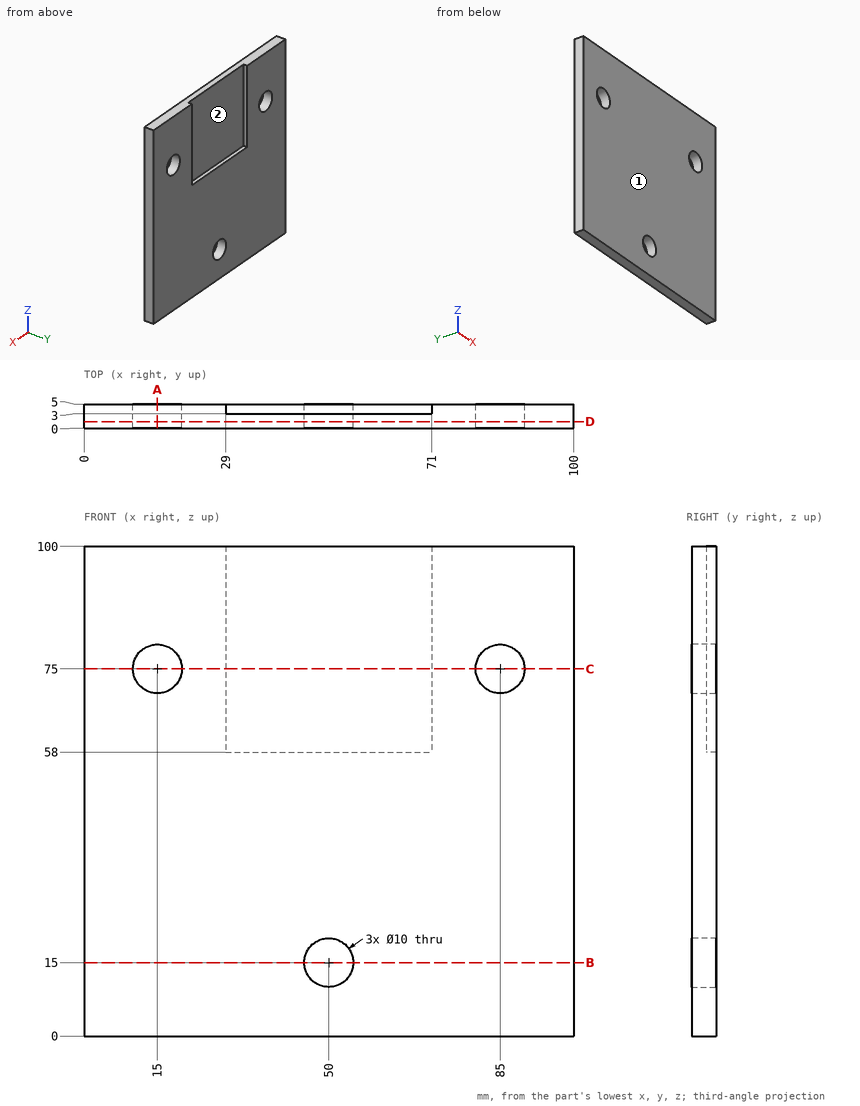
For this review, use the dimensioned drawing (mm, ordinates from the lowest corner) and the shaded views. Give positions to 0.01 mm unless a question says otherwise; leave off trailing zeros. Order: outer loops, then holes, each group sorted by start corner. A loop starts at its lowest first (then second) coordinate and runs counter-clockwise, first axis right, second up. Notation, with made-up numbers: (-38, -28) - (-3, -28) arc R12 ccw to (-3, -20) - close; hole circle Ø8 at (-9, 84). An arc over 180 degrees is marked (long way). Use CSV: the item, a comma, the result in double quotes. Start each with the question number.
Q1. Take a section at D-D (y = 1.4). State the section outline as (x, z) points, and give its area (3 significant figures).
Q2. Take a section at C-C (z = 75). State the section outline as (x, y) points, and give its area (3 significant figures).
Q3. Take a section at B-B (z = 15). State the section outline as (x, y) points, and give its area (3 significant figures).
Q4. For P1, Ø11.5, axis at x = 50, z = 15, coming from the -Y side; P2, Ø8, axis at x = 15, z = 75, coming from the -Y side; P3, Ø5, axis at x = 50.5, z = 65.5, coming from the +Y side; P4, Ø2, axis at x = 42, y = 4.5, coming from the +Z side, all flat-tipped, find the tip position at first contact; note any pin that passes through.
Q5. For line 1 (X direction, y = 1.3, z = 75); line 2 (X direction, y = 2.1, z = 15); line 3 (Y direction, x = 60, z = 76), list the stretches that pass through material, from the lowest coordinate up.
Q6. Take a section at A-A (x = 15). State the section outline as (y, z) points.
Q7. Draft analysis for pull direction X (two halves, no side actions). For the marked faces 1 and 2, state which applies: pulls with the +X half, pulls with the -X half, needs draft (parallel to the pull), parting line crosses it, or undercut.
Calculated:
1,outline,"(0, 0) - (100, 0) - (100, 100) - (0, 100) - close; hole circle Ø10 at (15, 75); hole circle Ø10 at (50, 15); hole circle Ø10 at (85, 75)"
1,area,"9,760 mm²"
2,outline,"(0, 0) - (10, 0) - (10, 5) - (0, 5) - close; (20, 0) - (80, 0) - (80, 5) - (71, 5) - (71, 3) - (29, 3) - (29, 5) - (20, 5) - close; (90, 0) - (100, 0) - (100, 5) - (90, 5) - close"
2,area,"316 mm²"
3,outline,"(0, 0) - (45, 0) - (45, 5) - (0, 5) - close; (55, 0) - (100, 0) - (100, 5) - (55, 5) - close"
3,area,"450 mm²"
4,P1,"stops at y = 0"
4,P2,"passes through"
4,P3,"stops at y = 3"
4,P4,"stops at z = 58"
5,line 1,"x = 0 to 10, 20 to 80, 90 to 100"
5,line 2,"x = 0 to 45, 55 to 100"
5,line 3,"y = 0 to 3"
6,outline,"(0, 0) - (5, 0) - (5, 70) - (0, 70) - close; (0, 80) - (5, 80) - (5, 100) - (0, 100) - close"
7,face 1,"needs draft"
7,face 2,"undercut"
